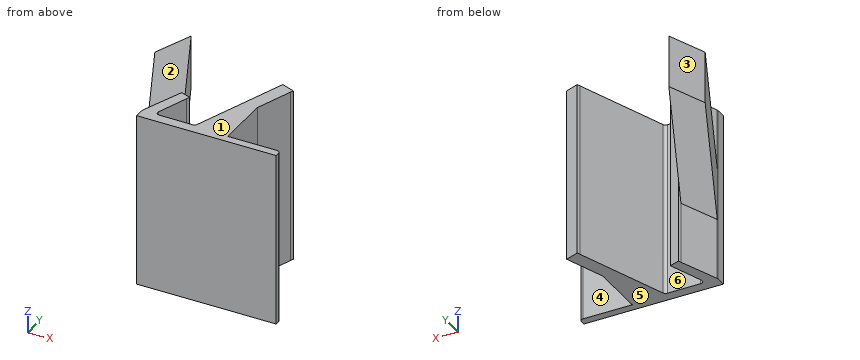
```python
from build123d import *

# Parameters (mm, degrees)
SALIENTE_EXTRUIR1_DEPTH = 50
CROQUIS3_W              = 15
CROQUIS3_H              = 12


with BuildPart() as part:
    # Croquis1 → Saliente-Extruir1 (new body)
    with BuildSketch(Plane.XY):
        with BuildLine():
            Line((-84.492533904, -6.921751872), (-44.492533904, -6.921751872))
            Line((-44.492533904, -6.921751872), (-44.492533904, -5.660932217))
            ThreePointArc((-44.492533904, -5.660932217), (-44.785427123, -4.953825435), (-45.492533904, -4.660932217))
            Line((-45.492533904, -4.660932217), (-59.602097354, -4.660932217))
            Line((-59.602097354, -4.660932217), (-59.602097354, 10.986403293))
            Line((-59.602097354, 10.986403293), (-55.79772825, 21.438821499))
            Line((-55.79772825, 21.438821499), (-55.455708107, 22.37851412))
            Line((-55.455708107, 22.37851412), (-59.21447859, 23.746594693))
            Line((-59.21447859, 23.746594693), (-59.556498733, 22.806902073))
            Line((-59.556498733, 22.806902073), (-69.073702494, -3.341400356))
            ThreePointArc((-69.073702494, -3.341400356), (-69.439818678, -3.818532257), (-70.013395115, -3.999380213))
            Line((-70.013395115, -3.999380213), (-79.590995067, -3.999380213))
            ThreePointArc((-79.590995067, -3.999380213), (-80.410147111, -3.572956649), (-80.530687688, -2.657360069))
            Line((-80.530687688, -2.657360069), (-77.297371662, 6.226102703))
            Line((-77.297371662, 6.226102703), (-76.955351518, 7.165795324))
            Line((-76.955351518, 7.165795324), (-79.774429381, 8.191855754))
            Line((-79.774429381, 8.191855754), (-80.129339821, 7.280632657))
            Line((-80.129339821, 7.280632657), (-84.424349875, -3.746691195))
            ThreePointArc((-84.424349875, -3.746691195), (-84.475340083, -3.924982082), (-84.492533904, -4.109622312))
            Line((-84.492533904, -4.109622312), (-84.492533904, -6.921751872))
        make_face()
    extrude(amount=SALIENTE_EXTRUIR1_DEPTH)

    # Barrer9: sweep along a path in Croquis7
    with BuildLine(Plane(origin=(-43.940534578, 17.114309903, -27.225418163), x_dir=(0.465907986, -0.181465559, -0.866025404), z_dir=(0.806976303, -0.314307567, 0.5))) as barrer9_path:
        Line((-60.30471847, -28.214335671), (-86.285480583, -13.214335671))
    # Croquis3 → Barrer9 (sweep)
    with BuildSketch(Plane(origin=(-72.036984482, 28.057539326, 0), x_dir=(0, 0, 1), z_dir=(-0.931815971, 0.362931117, 0))):
        with Locations((25, -28.214335671)):
            Rectangle(CROQUIS3_W, CROQUIS3_H)
    sweep(path=barrer9_path.line)


solid = part.part
```
Part model, mm, in its own coordinate system. Face numbers are marked on the shaded views. A direction names the side the tool comes from. Round coordinates to 2 decimals unless told otherwise and drop trailing zeros. Order: outer loops, then holes, each group sorted by start corner. A loop starts at its lowest first (then second) coordinate and runs counter-clockwise, first axis right, second up. Notation, with made-up numbers: M 68.5,63.25 L 125.5,63.25 A19 cw 125.5,84.25 Z; hole C -2.75,48 d2. An arc over 180 degrees is marked long. Answer in a Markdown table with one row per item. Add a question column.
Q1. Cut at C-C on z = 38. Give the cut face in (x, y).
Q2. Cut at D-D on x = -81.5. Give the cut face in (y, z).
Q3. Mould opens along X. For the marked faces 1, 2 and 3 say: +X half, -X half, draft (parallel to the pull), parting line (faces both ways), or undercut.
Q4. Wall check: L1, parallel to Y at x = -72.5, z = 14; L2, parallel to X at y = 4, z = 47; L3, parallel to X at y = 3.5, z = 22. Give the ranges that are in metal, low to high. Write a range as from..to.
Q5. Cut at A-A on z = 4.5. Give the cut face in (x, y), and give its area (3 significant figures).
Q6. Pin check, flat tips, straight feed: pin 1 (17 mm diameter, centred on y = 7, z = 19.5, fed in from +X); pin 2 (1 mm diameter, centred on y = 22.5, z = 19.5, fed in from -X); pin 3 (4 mm diameter, centred on y = 13.5, z = 15, fed in from -X); pin 4 (1.5 mm diameter, centred on x = -68.5, y = 3.5, fed in from +Z). Stop position of each tip, or through.
Q7. Cut at B-B on y = 17.5. Give the cut face in (x, z).
Q8. 3-axis set-ups, long thin cutter, end or side, ignore diameter. For the marked faces 4, 5 and 6: which of +Z, -Z, +X, -X, +Y, -Y reach the whole face in a straight line?
Established:
| question | item | result |
|---|---|---|
| 1 | outline | M -90.52,13.21 L -86.08,0.75 L -81.73,11.93 L -86.17,24.39 Z; M -84.49,-6.92 L -44.49,-6.92 L -44.49,-5.66 A1 ccw -45.49,-4.66 L -59.6,-4.66 L -59.6,10.99 L -55.46,22.38 L -59.21,23.75 L -69.07,-3.34 A1 cw -70.01,-4 L -79.59,-4 A1 cw -80.53,-2.66 L -76.96,7.17 L -79.77,8.19 L -84.42,-3.75 A1 ccw -84.49,-4.11 Z |
| 2 | outline | M -6.92,0 L 3.76,0 L 3.76,17.5 L 11.29,22.23 L 11.29,37.23 L 3.76,32.5 L 3.76,50 L -6.92,50 Z |
| 3 | face 1 | draft |
| 3 | face 2 | undercut |
| 3 | face 3 | -X half |
| 4 | L1 | y = -6.92..-4 |
| 4 | L2 | x = -81.41..-78.11, -66.4..-59.6 |
| 4 | L3 | x = -84.39..-78.29, -66.58..-59.6 |
| 5 | outline | M -84.49,-6.92 L -44.49,-6.92 L -44.49,-5.66 A1 ccw -45.49,-4.66 L -59.6,-4.66 L -59.6,10.99 L -55.46,22.38 L -59.21,23.75 L -69.07,-3.34 A1 cw -70.01,-4 L -79.59,-4 A1 cw -80.53,-2.66 L -76.96,7.17 L -79.77,8.19 L -84.42,-3.75 A1 ccw -84.49,-4.11 Z |
| 5 | area | 302 mm2 |
| 6 | pin 1 | stops at x = -57.96 |
| 6 | pin 2 | stops at x = -59.85 |
| 6 | pin 3 | stops at x = -63.67 |
| 6 | pin 4 | passes through |
| 7 | outline | M -90.09,40 L -83.71,29.71 L -83.71,44.71 L -90.09,55 Z; M -61.49,0 L -57.23,0 L -57.23,50 L -61.49,50 Z |
| 8 | face 4 | +Z, -Z, +X |
| 8 | face 5 | -Z, +X, -X, +Y, -Y |
| 8 | face 6 | +Z, -Z |
